Print and shaded views of the part. All mm, measured from the part's lowest x, y and z. A direction names the side the tool comes from. Coordinates: 2 decimals unless noted, no trailing zeros. Write each loop counter-clockwise with the first axis right and the second up, starting at its lowest first coordinate (ties: lowest second). Pieces come first, ordered by that corner, then holes. Notation, with made-up numbers: (73, 85.5) -> (109, 85.5) arc R20 cw to (109, 102.5) -> close; hole circle Ø6 at (43, -40). An arc over 180 degrees is marked (long way). Write item = value, one per line.
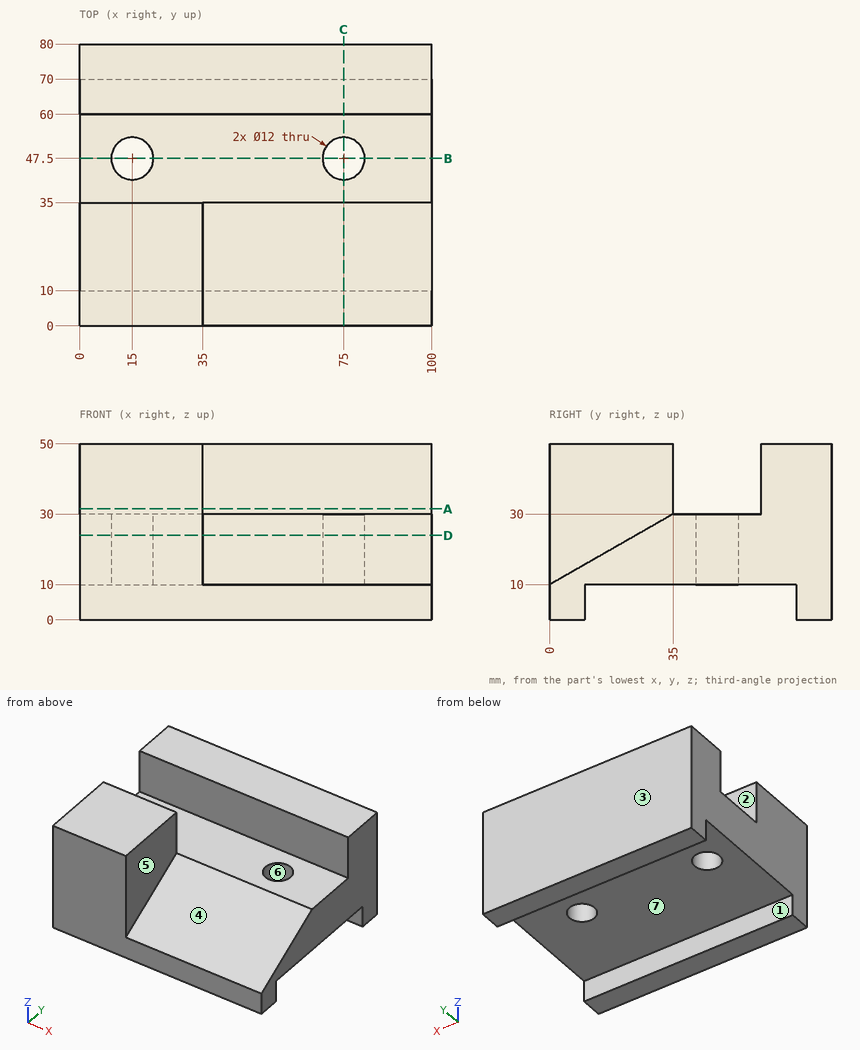
Q1. Saw through at A-A on z = 31.5. Give the cut face in (x, y).
Model answer:
outline = (0, 0) -> (35, 0) -> (35, 35) -> (0, 35) -> close; (0, 60) -> (100, 60) -> (100, 80) -> (0, 80) -> close
Q2. Saw through at D-D on z = 24. Give the cut face in (x, y), and give its area (3 significant figures).
Model answer:
outline = (0, 0) -> (35, 0) -> (35, 24.5) -> (100, 24.5) -> (100, 80) -> (0, 80) -> close; hole circle Ø12 at (15, 47.5); hole circle Ø12 at (75, 47.5)
area = 6,180 mm²
Q3. Mould opens along X. For the marked faces 5, 6 and 7 say: released by +X, released by -X, zero draft, split by the parting line, or undercut.
Model answer:
face_5 = released by +X
face_6 = undercut
face_7 = zero draft
Q4. Probe line 1 (Y direction, x = 15, z = 17); line 2 (X direction, y = 47, z = 19); line 3 (Y direction, x = 86.5, z = 4). List the from-to ranges inside material, lowest first. Write a range as from..to.
Model answer:
line_1 = 0..41.5, 53.5..80
line_2 = 0..9.02, 20.98..69.02, 80.98..100
line_3 = 0..10, 70..80
Q5. Pin check, flat tips, straight feed: pin 1 (15.5 mm diameter, centred on x = 75, y = 47.5, fed in from -Z); pin 2 (4 mm diameter, centred on x = 84.5, y = 23.5, fed in from +Z); pin 3 (10.5 mm diameter, centred on y = 10.5, z = 38.5, fed in from +X); pin 4 (6 mm diameter, centred on y = 36.5, z = 42, fed in from -X). Stop position of each tip, or through.
Model answer:
pin_1 = 10
pin_2 = 24.57
pin_3 = 35
pin_4 = 0
Q6. Saw through at C-C on x = 75. Give the cut face in (y, z).
Model answer:
outline = (0, 0) -> (10, 0) -> (10, 10) -> (41.5, 10) -> (41.5, 30) -> (35, 30) -> (0, 10) -> close; (53.5, 10) -> (70, 10) -> (70, 0) -> (80, 0) -> (80, 50) -> (60, 50) -> (60, 30) -> (53.5, 30) -> close
Q7. Saw through at B-B on y = 47.5. Give the cut face in (x, z), and give its area (3 significant figures).
Model answer:
outline = (0, 10) -> (9, 10) -> (9, 30) -> (0, 30) -> close; (21, 10) -> (69, 10) -> (69, 30) -> (21, 30) -> close; (81, 10) -> (100, 10) -> (100, 30) -> (81, 30) -> close
area = 1,520 mm²
Q8. Which spindle directions (+Z, -Z, +X, -X, +Y, -Y) get a long thin tool onto all of the face, cutting with end or side? Do the marked faces 1, 2, 3 and 4. Say none if no direction does.
Model answer:
face_1 = -Z, +X, -X
face_2 = +Z, +X, -X
face_3 = +Z, -Z, +X, -X, +Y
face_4 = +Z, +X, -Y
